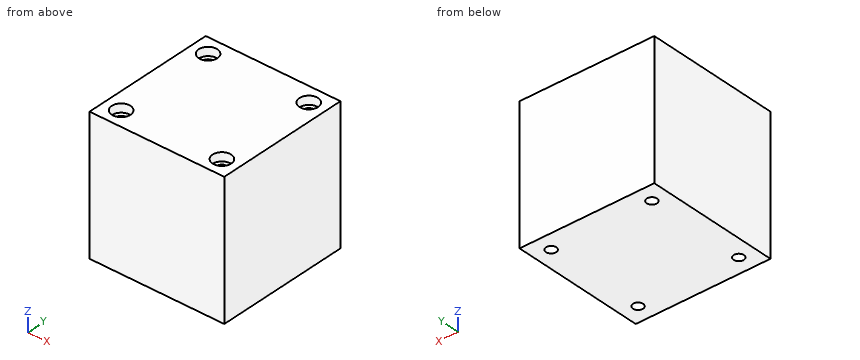
from build123d import *

# Parameters (mm, degrees)
SKETCH1_W                      = 31.75
SKETCH1_H                      = 31.75
BOSS_EXTRUDE1_DEPTH            = 31.75
CBORE_FOR_M2_SHCS1_D           = 2.4
CBORE_FOR_M2_SHCS1_CBORE_D     = 4.4
CBORE_FOR_M2_SHCS1_CBORE_DEPTH = 2


with BuildPart() as part:
    # Sketch1 → Boss-Extrude1 (new body)
    with BuildSketch(Plane.XY):
        Rectangle(SKETCH1_W, SKETCH1_H)
    extrude(amount=BOSS_EXTRUDE1_DEPTH)

    # CBORE for M2 SHCS1 (through all)
    with Locations(Plane.XY.offset(31.75)):
        with Locations((-11.875, 11.875), (11.875, 11.875), (11.875, -11.875), (-11.875, -11.875)):
            CounterBoreHole(CBORE_FOR_M2_SHCS1_D / 2, CBORE_FOR_M2_SHCS1_CBORE_D / 2, CBORE_FOR_M2_SHCS1_CBORE_DEPTH)


solid = part.part
Work out the finished part from the listing and answer in its coordinate system (mm). Round coordinates to 2 decimals unless told otherwise and drop trailing zeros. Loops run counter-clockwise (first coordinate to the right, second up) from the corner with the lowest first, then second, coordinate; pieces in that order, holes last. Notation, with made-up numbers: (10, -23) - (56, -23) arc R16 cw to (56, -2) - close; hole circle Ø11 at (38, 31). An arc over 180 degrees is marked (long way). Use one line per item in the form item = value. Start each with the question number.
(1) Find section A-A on x = 11.5. Determine the outline of the cut face in (y, z) (3 decimals), and give its area (3 significant figures).
(2) Find section B-B on z = 26. Determine the outline of the cut face in (x, y) (3 decimals).
(3) Find section C-C on x = -12.5. Determine the outline of the cut face in (y, z) (3 decimals), and give its area (3 significant figures).
(4) Flat-ended cylindrical pins translate along their axes: P1, Ø1.9, axis at x = -11.875, y = 11.875, coming from the -Z side; P2, Ø3, axis at x = 11.875, y = 11.875, coming from the +Z side; P3, Ø5.5, axis at x = 11.875, y = 11.875, coming from the +Z side. Find the tip coordinate at first contact, or state that the pin passes through.
(5) Consider line 1 (X direction, y = 12, z = 19.5) (3 decimals); line 2 (X direction, y = 11.5, z = 12) (3 decimals); line 3 (Z direction, x = 13.5, y = -13). Determine where each line is inside the solid, lowest interval first.
Answer list:
q1.outline = (-15.875, 0) - (-13.015, 0) - (-13.015, 29.75) - (-14.043, 29.75) - (-14.043, 31.75) - (-15.875, 31.75) - close; (-10.735, 0) - (10.735, 0) - (10.735, 29.75) - (9.707, 29.75) - (9.707, 31.75) - (-9.707, 31.75) - (-9.707, 29.75) - (-10.735, 29.75) - close; (13.015, 0) - (15.875, 0) - (15.875, 31.75) - (14.043, 31.75) - (14.043, 29.75) - (13.015, 29.75) - close
q1.area = 855 mm^2
q2.outline = (-15.875, -15.875) - (15.875, -15.875) - (15.875, 15.875) - (-15.875, 15.875) - close; hole circle Ø2.4 at (-11.875, -11.875); hole circle Ø2.4 at (-11.875, 11.875); hole circle Ø2.4 at (11.875, -11.875); hole circle Ø2.4 at (11.875, 11.875)
q3.outline = (-15.875, 0) - (-12.899, 0) - (-12.899, 29.75) - (-13.984, 29.75) - (-13.984, 31.75) - (-15.875, 31.75) - close; (-10.851, 0) - (10.851, 0) - (10.851, 29.75) - (9.766, 29.75) - (9.766, 31.75) - (-9.766, 31.75) - (-9.766, 29.75) - (-10.851, 29.75) - close; (12.899, 0) - (15.875, 0) - (15.875, 31.75) - (13.984, 31.75) - (13.984, 29.75) - (12.899, 29.75) - close
q3.area = 869 mm^2
q4.P1 = through
q4.P2 = 29.75
q4.P3 = 31.75
q5.line_1 = -15.875 to -13.068, -10.682 to 10.682, 13.068 to 15.875
q5.line_2 = -15.875 to -13.015, -10.735 to 10.735, 13.015 to 15.875
q5.line_3 = 0 to 29.75
